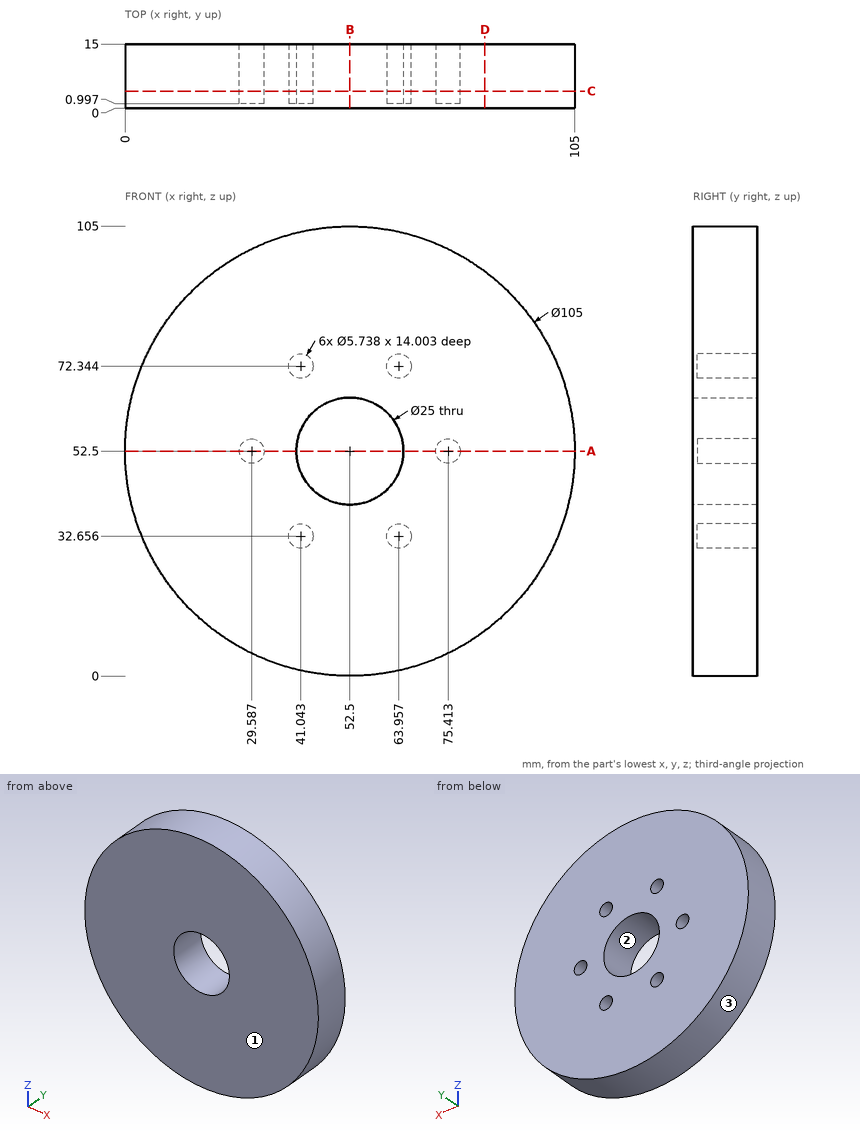
Print and shaded views of the part. All mm, measured from the part's lowest x, y and z. Round coordinates to 2 decimals unless told otherwise and drop trailing zeros. Write each loop counter-clockwise with the first axis right and the second up, starting at its lowest first coordinate (ties: lowest second). Pieces come first, ordered by that corner, then holes. Notation, with made-up numbers: (35.5, 29) - (39.5, 29) arc R26 ccw to (39.5, 68) - close; hole circle Ø11 at (0, 89). An arc over 180 degrees is marked (long way). Write each question's results on one line, items separated by ' | '. Start each with the question number.
Item 1: Saw through at C-C (y = 4). Write the cut outline in (x, z) (1 decimal), and give its area (3 significant figures).
Item 2: Drop flat-ended pins along their axis: P1, Ø2, axis at y = 8.5, z = 68, coming from the +X side; P2, Ø4, axis at x = 63, y = 7.5, coming from the -Z side; P3, Ø1.7, axis at x = 74.5, z = 54, coming from the +Y side; P4, Ø20, axis at x = 52.5, z = 52.5, coming from the +Y side. Give the stop position or say it passes through.
Item 3: Saw through at B-B (x = 52.5). Write the cut outline in (y, z).
Item 4: Saw through at D-D (x = 84). Write the cut outline in (y, z), and give its area (3 significant figures).
Item 5: Saw through at A-A (z = 52.5). Write the cut outline in (x, y) (1 decimal), and give its area (3 significant figures).
Item 6: Mould opens along Z. For the marked faces 1, 2 and 3 say: pulls with the +Z half, pulls with the -Z half, needs draft (parallel to the pull), parting line crosses it, or undercut.
Item 7: Wall check: L1, parallel to X at y = 4, z = 52.5 (1 decimal); L2, parallel to Z at x = 39.5, y = 9.75 (1 decimal); L3, parallel to X at y = 11.75, z = 70 (1 decimal). Give the ranges that are in metal, low to high. Write a range as [from, to].
Results are:
1) outline: circle Ø105 at (52.5, 52.5); hole circle Ø5.7 at (29.6, 52.5); hole circle Ø5.7 at (41, 32.7); hole circle Ø5.7 at (41, 72.3); hole circle Ø25 at (52.5, 52.5); hole circle Ø5.7 at (64, 32.7); hole circle Ø5.7 at (64, 72.3); hole circle Ø5.7 at (75.4, 52.5) | area: 8,010 mm²
2) P1: stops at x = 102.96 | P2: stops at z = 0.69 | P3: stops at y = 1 | P4: passes through
3) outline: (0, 0) - (15, 0) - (15, 40) - (0, 40) - close; (0, 65) - (15, 65) - (15, 105) - (0, 105) - close
4) outline: (0, 10.5) - (15, 10.5) - (15, 94.5) - (0, 94.5) - close | area: 1,260 mm²
5) outline: (0, 0) - (40, 0) - (40, 15) - (32.5, 15) - (32.5, 1) - (26.7, 1) - (26.7, 15) - (0, 15) - close; (65, 0) - (105, 0) - (105, 15) - (78.3, 15) - (78.3, 1) - (72.5, 1) - (72.5, 15) - (65, 15) - close | area: 1,040 mm²
6) face 1: needs draft | face 2: undercut | face 3: parting line crosses it
7) L1: x = [0, 26.7], [32.5, 40], [65, 72.5], [78.3, 105] | L2: z = [1.6, 30.2], [35.1, 69.9], [74.8, 103.4] | L3: x = [3, 39.4], [42.7, 62.3], [65.6, 102]
